For this review, take the finished solid that the model builds, in its own axes (mm). A direction names the side the tool comes from. Coordinates: 2 decimals unless noted, no trailing zeros. Loops run counter-clockwise (first coordinate to the right, second up) from the corner with the lowest first, then second, coordinate; pieces in that order, holes last. Notation, with made-up numbers: M -39.75,29.25 L -8.75,29.25 A19 ccw -8.75,57.25 Z; hole C 55.25,61.5 d1. An arc over 180 degrees is marked long. Use one line per item in the form item = value.
```python
from build123d import *

# Parameters (mm, degrees)
F0_W     = 75.3582566977
F0_H     = 34.1903194785
F0_W_2   = 75.8234262466
F0_H_2   = 70.0087472796
F0_H_3   = 58.2362934947
F1_DEPTH = 76.2
F2_DEPTH = 30
F3_R     = 20
F4_SIZE  = 5.08
F5_R     = 5.08
F6_R     = 8.6494969127
F6_R_2   = 7.8863164194
F6_R_3   = 9.4186807379
F7_DEPTH = 204.6777398715


with BuildPart() as f1:
    # F0 (on Front) → F1 (new body)
    with BuildSketch(Plane.XZ):
        Polygon((-75.3582566977, -34.1903194785), (-75.3582566977, -76.0560184717), (75.8234262466, -76.0560184717), (75.8234262466, -34.1903194785), (0, -34.1903194785), align=None)
        Polygon((-75.3582566977, -76.4316990972), (-75.3582566977, -76.0560184717), (-75.3582566977, -34.1903194785), (-75.3582566977, 0), (-168.3024764061, 0), (-168.3024764061, -76.4316990972), align=None)
        with Locations((-37.6791283488, -17.0951597393)):
            Rectangle(F0_W, F0_H)
        with Locations((37.9117131233, -17.0951597393)):
            Rectangle(F0_W_2, F0_H)
        with Locations((-37.6791283488, 35.0043736398)):
            Rectangle(F0_W, F0_H_2)
        with Locations((37.9117131233, 35.0043736398)):
            Rectangle(F0_W_2, F0_H_2)
        with Locations((37.9117131233, 99.126894027)):
            Rectangle(F0_W_2, F0_H_3)
    extrude(amount=F1_DEPTH)

    # F0 (on Front) → F2 (join)
    with BuildSketch(Plane.XZ):
        Polygon((-75.3582566977, -34.1903194785), (-75.3582566977, -76.0560184717), (75.8234262466, -76.0560184717), (75.8234262466, -34.1903194785), (0, -34.1903194785), align=None)
        Polygon((-75.3582566977, -76.4316990972), (-75.3582566977, -76.0560184717), (-75.3582566977, -34.1903194785), (-75.3582566977, 0), (-168.3024764061, 0), (-168.3024764061, -76.4316990972), align=None)
        with Locations((-37.6791283488, -17.0951597393)):
            Rectangle(F0_W, F0_H)
        with Locations((37.9117131233, -17.0951597393)):
            Rectangle(F0_W_2, F0_H)
        with Locations((-37.6791283488, 35.0043736398)):
            Rectangle(F0_W, F0_H_2)
        with Locations((37.9117131233, 35.0043736398)):
            Rectangle(F0_W_2, F0_H_2)
        with Locations((37.9117131233, 99.126894027)):
            Rectangle(F0_W_2, F0_H_3)
    extrude(amount=F2_DEPTH)

    # F3
    f3_edges = [f1.edges().sort_by_distance(p)[0] for p in [
        (0, -38.1, 128.245041),
        (-75.358257, -38.1, 70.008747),
        (-168.302476, -38.1, 0),
    ]]
    fillet(f3_edges, radius=F3_R)

    # F4
    f4_edges = [f1.edges().sort_by_distance(p)[0] for p in [
        (47.911713, -76.2, 128.245041),
        (5.857864, -76.2, 122.387176),
        (75.823426, -76.2, 26.094511),
        (0, -76.2, 89.126894),
        (0.232585, -76.2, -76.056018),
        (-27.679128, -76.2, 70.008747),
        (-75.358257, -76.2, -76.243859),
        (-69.500392, -76.2, 64.150883),
        (-121.830367, -76.2, -76.431699),
        (-75.358257, -76.2, 25.004374),
        (-168.302476, -76.2, -48.21585),
        (-111.830367, -76.2, 0),
        (-162.444612, -76.2, -5.857864),
    ]]
    chamfer(f4_edges, length=F4_SIZE)

    # F5
    f5_edges = [f1.edges().sort_by_distance(p)[0] for p in [
        (47.911713, 0, 128.245041),
        (5.857864, 0, 122.387176),
        (75.823426, 0, 26.094511),
        (0, 0, 89.126894),
        (0.232585, 0, -76.056018),
        (-27.679128, 0, 70.008747),
        (-75.358257, 0, -76.243859),
        (-69.500392, 0, 64.150883),
        (-121.830367, 0, -76.431699),
        (-75.358257, 0, 25.004374),
        (-168.302476, 0, -48.21585),
        (-111.830367, 0, 0),
        (-162.444612, 0, -5.857864),
    ]]
    fillet(f5_edges, radius=F5_R)

    # F6 (on face) → F7 (cut, through all)
    with BuildSketch(Plane.XY.offset(128.2450407743)):
        with Locations((-113.8509809971, -35.9056405723)):
            Circle(F6_R)
        with Locations((-28.7020821124, -35.6748849154)):
            Circle(F6_R_2)
        with Locations((45.8320491016, -35.9056405723)):
            Circle(F6_R_3)
    extrude(amount=-F7_DEPTH, mode=Mode.SUBTRACT)


solid = f1.part
```
1. Wall thickness on line 1 along X through (y, z) = (-36.5, -22.5); line 2 along X through (y, z) = (-45.5, 47); line 3 along Z through (x, y) = (19, -38): over which ranges is each line inside the solid? List them lowest first. Write a range as from..to.
Computed values:
line_1 = -168.3..-122.48, -105.22..-36.55, -20.86..36.43, 55.23..75.82
line_2 = -75.36..75.82
line_3 = -76.06..128.22
2. Consider section D-D on z = 9. Write out the cut boundary in (x, y).
Computed values:
outline = M -75.36,-71.12 L -70.28,-76.2 L 70.74,-76.2 L 75.82,-71.12 L 75.82,-5.08 A5.08 ccw 70.74,0 L -70.28,0 A5.08 ccw -75.36,-5.08 Z; hole C -28.7,-35.67 d15.77; hole C 45.83,-35.91 d18.84
3. Consider section A-A on y = -39. Write out the cut boundary in (x, z).
Computed values:
outline = M -168.3,-76.43 L -121.93,-76.43 L -121.93,0 L -148.3,0 A20 ccw -168.3,-20 Z; M -105.77,-76.43 L -75.36,-76.43 L -75.36,-76.06 L -35.85,-76.06 L -35.85,70.01 L -55.36,70.01 A20 ccw -75.36,50.01 L -75.36,0 L -105.77,0 Z; M -21.55,-76.06 L 36.94,-76.06 L 36.94,128.25 L 20,128.25 A20 ccw 0,108.25 L 0,70.01 L -21.55,70.01 Z; M 54.73,-76.06 L 75.82,-76.06 L 75.82,128.25 L 54.73,128.25 Z
4. Tool access review of faces 5 (the face through (-3.401, -73.624, -73.552)), 6 (the face through (-27, -45, 70.009)), 7 (the face through (-73.83, -1.45, 22.08)): name each direction out of +Z, -Z, +X, -X, +Y, -Y from which nothing blocks a thin tool from reaching the whole face with its end or side.
Computed values:
face_5 = -Z, +X, -Y
face_6 = +Z, -X, +Y, -Y
face_7 = +Z, -X, +Y
5. For pin 1 Ø16.5 at (x, y) = (-16.5, -39) entering from +Z; pin 2 Ø6 at (y, z) = (-17.5, 61.5) entering from -X; pin 3 Ø1 at (x, y) = (-124.5, -41) entering from +Z; pin 4 Ø2 at (x, z) = (-77.5, 47.5) entering from -Y, all flat-tipped, find the tip position at first contact; note any pin that passes through.
Computed values:
pin_1 = 70.01
pin_2 = -73.47
pin_3 = 0
pin_4 = through
6. Consider section C-C on z = 86. Write out the cut boundary in (x, y).
Computed values:
outline = M 0,-71.12 L 5.08,-76.2 L 70.74,-76.2 L 75.82,-71.12 L 75.82,-5.08 A5.08 ccw 70.74,0 L 5.08,0 A5.08 ccw 0,-5.08 Z; hole C 45.83,-35.91 d18.84
7. Consider section B-B on x = -135.5. Write out the cut boundary in (y, z), plus the area to 3 significant figures.
Computed values:
outline = M -76.2,-71.35 L -71.12,-76.43 L -5.08,-76.43 A5.08 ccw 0,-71.35 L 0,-5.08 A5.08 ccw -5.08,0 L -71.12,0 L -76.2,-5.08 Z
area = 5,790 mm2
8. Draft analysis for pull direction X (two halves, no side actions). For faces 1 (the face through (-168.302, -38, -48)), 2 (the face through (-111, -45, 0)), 3 (the face through (-122.492, -35.525, -37.681)), 4 (the face through (-77.886, -73.648, -73.717)), state which applies: +X half, -X half, draft (parallel to the pull), parting line (faces both ways), or undercut.
Computed values:
face_1 = -X half
face_2 = draft
face_3 = undercut
face_4 = +X half
